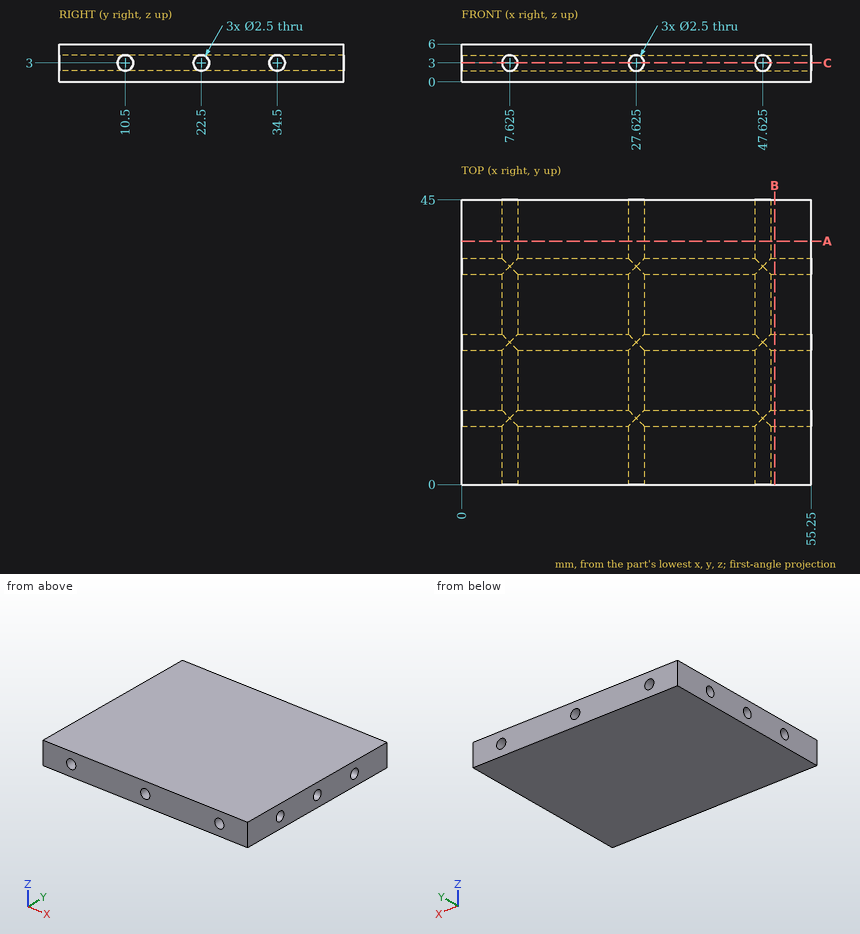
The figure shows three views and two pictorial views of one solid part (mm, origin at its lowest corner). Answer the questions. Give positions to 0.01 mm unless a question says otherwise; leave off trailing zeros. Loops run counter-clockwise (first coordinate to the right, second up) from the corner with the lowest first, then second, coordinate; pieces in that order, holes last. Notation, with made-up numbers: M -14,50.5 L 39,50.5 A25 ccw 39,62.5 Z; hole C 18,-5 d3. An arc over 180 degrees is marked long. Write each question's results on one line, items separated by ' | '.
1. Section B-B on x = 49.5 is taken. Give the vertices of the cut face in (y, z), plus the area to 3 significant figures.
Values:
outline: M 0,0 L 45,0 L 45,6 L 0,6 Z; hole C 10.5,3 d2.5; hole C 22.5,3 d2.5; hole C 34.5,3 d2.5 | area: 255 mm^2
2. Straight lines are drawn through the part: line 1 (Y direction, x = 53.5, z = 3); line 2 (X direction, y = 16.5, z = 3.1); line 3 (X direction, y = 25, z = 3.35) (3 decimals). For each, find the intervals that lie inside material, in ascending order. Write a range as [from, to].
Values:
line 1: y = [0, 9.25], [11.75, 21.25], [23.75, 33.25], [35.75, 45] | line 2: x = [0, 6.38], [8.87, 26.38], [28.87, 46.38], [48.87, 55.25] | line 3: x = [0, 6.425], [8.825, 26.425], [28.825, 46.425], [48.825, 55.25]
3. Section C-C on z = 3 is taken. State how many separate pieces and enclosed holes the cut face has, plus the area to 3 significant figures.
Values:
separate pieces: 16 | enclosed holes: 0 | area: 1,790 mm^2
4. Section A-A on y = 38.5 is taken. Give the vertices of the cut face in (x, z) (3 decimals), plus the area to 3 significant figures.
Values:
outline: M 0,0 L 55.25,0 L 55.25,6 L 0,6 Z; hole C 7.625,3 d2.5; hole C 27.625,3 d2.5; hole C 47.625,3 d2.5 | area: 317 mm^2
